Read the model definition and answer for the solid it produces. Units are mm, in the model's axes. Face numbers are marked on the shaded views. A direction names the side the tool comes from. Coordinates: 2 decimals unless noted, no trailing zeros. Write each loop counter-clockwise with the first axis right and the second up, starting at its lowest first coordinate (ties: lowest second). Pieces come first, ordered by that corner, then holes. Notation, with made-up numbers: M -5,-4.5 L 35,-4.5 A18 ccw 35,8.5 Z; hole C 9.25,-3 d1. An arc over 180 degrees is marked long. Write item = value, one per line.
from build123d import *

# Parameters (mm, degrees)
SKETCH4_R               = 9.525
F_1ST_BOLT_HOLE_DEPTH   = 20.05
BOLT_HOLE_PATTERN_COUNT = 4


with BuildPart() as part:
    # Sketch3 → Base-Revolve (revolve)
    with BuildSketch(Plane.XY):
        with BuildLine():
            Line((26.2509, 61.9125), (26.2509, -1.5875))
            Line((26.2509, -1.5875), (46.0375, -1.5875))
            Line((46.0375, -1.5875), (46.0375, 0))
            Line((46.0375, 0), (76.2, 0))
            Line((76.2, 0), (76.2, 17.4625))
            Line((76.2, 17.4625), (41.377092519, 17.4625))
            ThreePointArc((41.377092519, 17.4625), (39.421017335, 18.13662118), (38.295576299, 19.872723702))
            Line((38.295576299, 19.872723702), (30.31948378, 52.010825428))
            ThreePointArc((30.31948378, 52.010825428), (30.2494576, 52.390367381), (30.226, 52.775601727))
            Line((30.226, 52.775601727), (30.226, 61.9125))
            Line((30.226, 61.9125), (26.2509, 61.9125))
        make_face()
    revolve(axis=Axis((0, 0, 0), (0, 1, 0)))

    # Sketch4 → 1st Bolt Hole (cut, through all)
    with BuildSketch(Plane(origin=(0, 17.4625, 0), x_dir=(-1, 0, 0), z_dir=(0, 1, 0))):
        with Locations((-42.656216575, 42.656216575)):
            Circle(SKETCH4_R)
    f_1st_bolt_hole = extrude(amount=-F_1ST_BOLT_HOLE_DEPTH, mode=Mode.SUBTRACT)

    # Bolt Hole Pattern: 1st Bolt Hole ×4 about axis
    bolt_hole_pattern_axis = Axis((0, 0, 0), (0, 1, 0))
    for i in range(1, BOLT_HOLE_PATTERN_COUNT):
        add(f_1st_bolt_hole.rotate(bolt_hole_pattern_axis, i * 360 / BOLT_HOLE_PATTERN_COUNT), mode=Mode.SUBTRACT)


solid = part.part
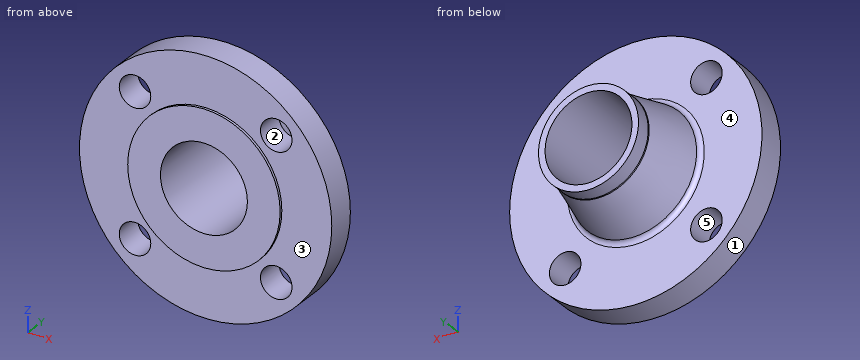
Item 1: For a pull along Z with two mould halves and no side action, classify the marked faces 1, 2 and 3 as released by +Z, released by -Z, zero draft, split by the parting line, or undercut.
Worked answers:
face_1 = split by the parting line
face_2 = undercut
face_3 = zero draft
Item 2: Find section D-D (x = 56). Determine the outline of the cut face in (y, z).
Worked answers:
outline = M 0,-51.68 L 17.46,-51.68 L 17.46,51.68 L 0,51.68 Z
Item 3: Consider line 1 along X through (y, z) = (14, 0); line 2 along Y through (x, z) = (-41, -20); line 3 along Y through (x, z) = (55, 14). Determine where each line is inside the solid, lowest interval first. Write a range as from..to.
Worked answers:
line_1 = -76.2..-26.25, 26.25..76.2
line_2 = -1.59..17.46
line_3 = 0..17.46
Item 4: Which of the six approach directions +Z, -Z, +X, -X, +Y, -Y give full straight-line access (tool end or side, diameter ignored) to the marked faces 4 and 5?
Worked answers:
face_4 = +Y
face_5 = +Y, -Y
Item 5: Flat-ended cylindrical pins translate along their axes: pin 1 (4 mm diameter, centred on y = 35.5, z = 10.5, fed in from +X); pin 2 (8 mm diameter, centred on x = 32.5, z = -42.5, fed in from +Y); pin 3 (6 mm diameter, centred on y = 13, z = -12.5, fed in from -X). Find the tip coordinate at first contact, or state that the pin passes through.
Worked answers:
pin_1 = 33.56
pin_2 = 17.46
pin_3 = -75.61
Item 6: Find section C-C (y = 40). Determine the outline of the cut face in (x, z).
Worked answers:
outline = C 0,0 d66.6; hole C 0,0 d52.5
